Can you work these out from the model? Positions are in its coordinate system, mm. Face numbers are marked on the shaded views. A direction names the side the tool comes from. Round coordinates to 2 decimals unless told otherwise and drop trailing zeros. Order: outer loops, then holes, each group sorted by start corner. A loop starts at its lowest first (then second) coordinate and runs counter-clockwise, first axis right, second up. Notation, with made-up numbers: M 0.5,84 L 55.5,84 A16 cw 55.5,109 Z; hole C 4.5,15.25 d3. An arc over 180 degrees is marked long. Answer as a JSON object with one key per item and string values. Group by question number.
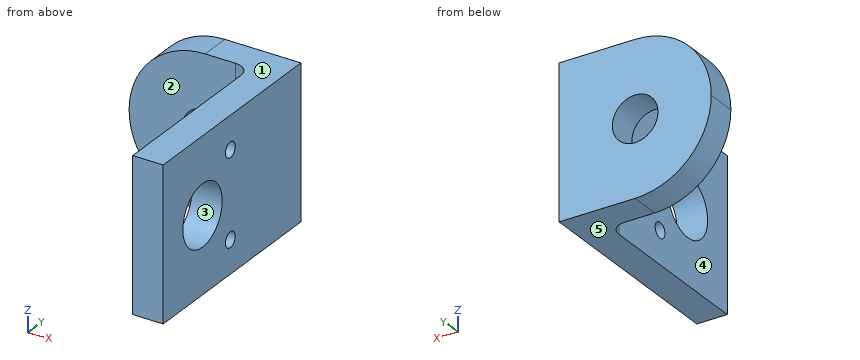
Autodesk Inventor part; units mm, degrees
ref_plane "YZ Plane" through (0, 0, 0) normal (1, 0, 0) x (0, 1, 0)
ref_plane "XZ Plane" through (0, 0, 0) normal (0, 1, 0) x (-1, 0, 0)
ref_plane "XY Plane" through (0, 0, 0) normal (0, 0, 1) x (1, 0, 0)
sketch "Sketch1" plane through (0, 0, 0) normal (0, 0, 1) x (1, 0, 0)
  line L0 (0, 0) -> (0, 34.925)
  line L1 (-3.175, 38.1) -> (-25.4, 38.1)
  line L2 (-25.4, 38.1) -> (-25.4, 44.45)
  line L3 (-25.4, 44.45) -> (6.35, 44.45)
  line L4 (6.35, 44.45) -> (6.35, 0)
  line L5 (6.35, 0) -> (0, 0)
  arc A0 (0, 34.925) -> (-3.175, 38.1) centre (-3.175, 34.925) ccw
  point P0 (0, 38.1)
  dimension "d0" = 6.35
  dimension "d1" = 38.1
  dimension "d2" = 25.4
  dimension "d3" = 3.175
extrude "Extrusion1" add sketch "Sketch1" along normal blind 31.75
sketch "Sketch2" plane through (6.35, 0, 0) normal (1, 0, 0) x (0, 0, -1)
  line L0 (0, 38.1) -> (-31.75, 38.1) construction
  line L1 (0, 0) -> (-31.75, 0) construction
  line L2 (-15.875, 38.1) -> (-15.875, 0) construction
  line L3 (0, 0) -> (-31.75, 0) construction
  circle A0 centre (-15.875, 12.7) radius 6.35
  line L4 (0, 44.45) -> (-31.75, 44.45) construction
  line L5 (-15.875, 12.7) -> (-31.75, 28.575) construction
  line L6 (-31.75, 0) -> (-31.75, 44.45) construction
  circle A1 centre (-24.8553, 21.6803) radius 1.5875
  circle A2 centre (-6.8947, 21.6803) radius 1.5875
  dimension "d15" = 12.7
  dimension "d21" = 31.75
  dimension "d25" = 45
  dimension "d26" = 3.175
  dimension "d27" = 12.7
extrude "Extrusion2" cut sketch "Sketch2" against normal through all
sketch "Sketch3" plane through (-25.4, 44.45, 0) normal (0, 1, 0) x (1, 0, 0)
  line L0 (0, 0) -> (0, -31.75) construction
  line L1 (0, 0) -> (0, -31.75) construction
  line L2 (0, -15.875) -> (15.875, -15.875) construction
  circle A0 centre (15.875, -15.875) radius 4.7625
  dimension "d17" = 9.525
  dimension "d18" = 15.875
extrude "Extrusion3" cut sketch "Sketch3" against normal through all
fillet "Fillet1" radius 15.875 2 edges at (-25.4, 41.275, 31.75) (-25.4, 41.275, 0)
equation "\"d7\" = d6"
properties part number "Corner Hinge"
1) Which directions (+Z, -Z, +X, -X, +Y, -Y) give clear straight access to the entire face, cutting with the end or side of a thin tool? Please do the marked faces 1 and 2.
2) If we section it at A-A on y = 12.7: Write out the boundary of the cut face in (x, z) (3 decimals), plus the area to 3 significant figures.
3) If we section it at D-D on z = 16.5: Write out the boundary of the cut face in (x, y) (3 decimals).
4) If we section it at C-C on z = 10.5: Write out the boundary of the cut face in (x, y) (3 decimals).
5) I need wall thicknesses on line 1 along Y through (x, z) = (-13, 10.5); line 2 along X through (y, z) = (32, 29); line 3 along Y through (x, z) = (4, 8). Which ranges of each line are inside material? Lowest first, please.
6) If we section it at B-B on x = -6.5: Write out the boundary of the cut face in (y, z).
7) For pin 1 (1 mm diameter, centred on x = -1.5, z = 25, fed in from -Y); pin 2 (18 mm diameter, centred on x = -16, z = 14.5, fed in from -Y), each with a flat end and sliding along its axis, tell me the tip position at first contact or that it passes through.
8) We'd pull the mould along Z, two halves only. Please class the marked faces 3, 4 and 5: +Z half, -Z half, draft (parallel to the pull), parting line (faces both ways), or undercut.
Findings:
{
 "1": {"face 1": "+Z, +X, -X, +Y, -Y", "face 2": "+Z, -Z, -X, -Y"},
 "2": {"outline": "M 0,0 L 6.35,0 L 6.35,9.525 L 0,9.525 Z; M 0,22.225 L 6.35,22.225 L 6.35,31.75 L 0,31.75 Z", "area": "121 mm^2"},
 "3": {"outline": "M -25.388,38.1 L -14.246,38.1 L -14.246,44.45 L -25.388,44.45 Z; M -4.804,38.1 L -3.175,38.1 A3.175 cw 0,34.925 L 0,19.019 L 6.35,19.019 L 6.35,44.45 L -4.804,44.45 Z; M 0,0 L 6.35,0 L 6.35,6.381 L 0,6.381 Z"},
 "4": {"outline": "M -24.462,38.1 L -3.175,38.1 A3.175 cw 0,34.925 L 0,16.081 L 6.35,16.081 L 6.35,44.45 L -24.462,44.45 Z; M 0,0 L 6.35,0 L 6.35,9.319 L 0,9.319 Z"},
 "5": {"line 1": "y = 38.1 to 44.45", "line 2": "x = 0 to 6.35", "line 3": "y = 0 to 20.54, 22.82 to 44.45"},
 "6": {"outline": "M 38.1,0 L 44.45,0 L 44.45,12.2 L 38.1,12.2 Z; M 38.1,19.55 L 44.45,19.55 L 44.45,31.75 L 38.1,31.75 Z"},
 "7": {"pin 1": "stops at y = 37.24", "pin 2": "stops at y = 38.1"},
 "8": {"face 3": "undercut", "face 4": "draft", "face 5": "-Z half"}
}
